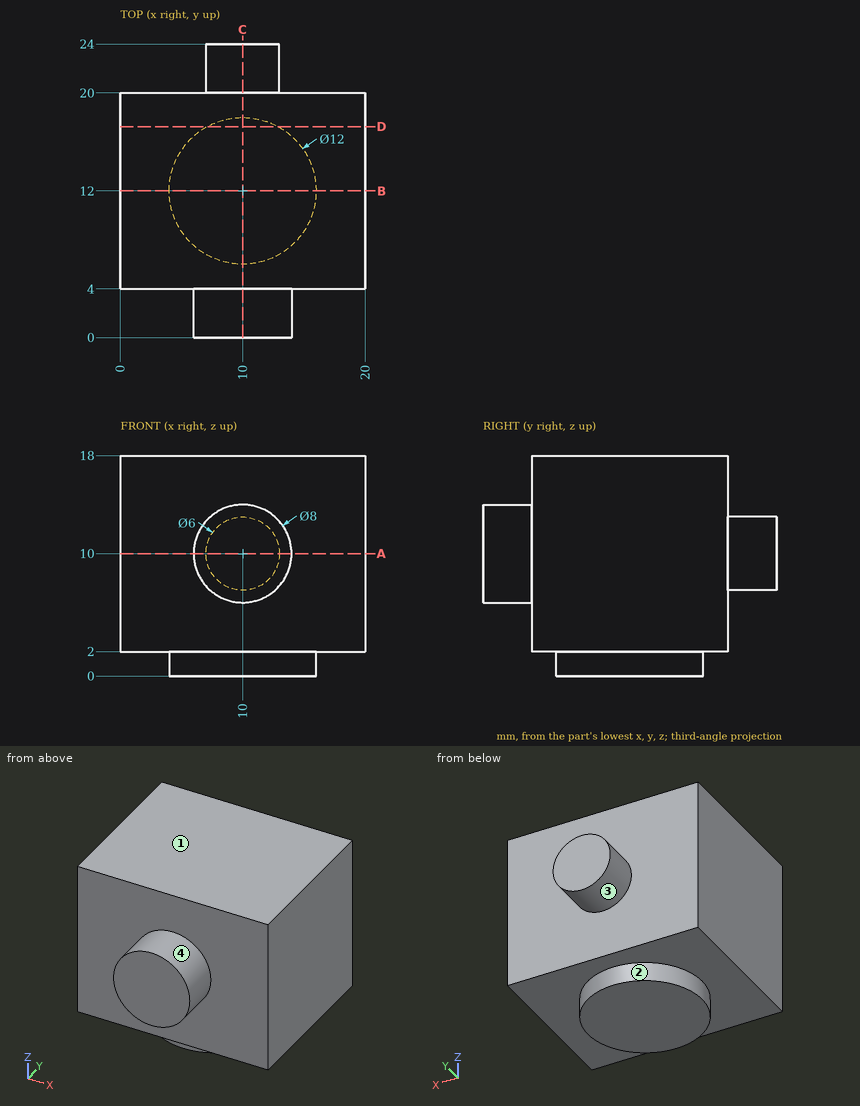
Design review of the part shown in the three views and the two pictorial views. Dimensions are in mm from the part's minimum x, y and z. A direction names the side the tool comes from. Coordinates: 2 decimals unless noted, no trailing zeros. Loops run counter-clockwise (first coordinate to the right, second up) from the corner with the lowest first, then second, coordinate; pieces in that order, holes last.
Q1. Tool access review of the marked faces 1, 2, 3 and 4: name each direction out of +Z, -Z, +X, -X, +Y, -Y from which nothing blocks a thin tool from reaching the whole face with its end or side.
Reported:
face 1: +Z, +X, -X, +Y, -Y
face 2: -Z
face 3: +Y
face 4: -Y
Q2. For pin 1 (4 mm diameter, centred on x = 9.5, z = 2, fed in from +Y), flat-tipped, find the tip position at first contact; note if it passes through.
Reported:
pin 1: stops at y = 20
Q3. We need section A-A on z = 10. State the section outline as (x, y) points.
Reported:
outline: (0, 4) - (6, 4) - (6, 0) - (14, 0) - (14, 4) - (20, 4) - (20, 20) - (13, 20) - (13, 24) - (7, 24) - (7, 20) - (0, 20) - close
Q4. We need section B-B on y = 12. State the section outline as (x, z) points, and give its area (3 significant figures).
Reported:
outline: (0, 2) - (4, 2) - (4, 0) - (16, 0) - (16, 2) - (20, 2) - (20, 18) - (0, 18) - close
area: 344 mm2
Q5. We need section D-D on y = 17.25. State the section outline as (x, z) points.
Reported:
outline: (0, 2) - (7.1, 2) - (7.1, 0) - (12.9, 0) - (12.9, 2) - (20, 2) - (20, 18) - (0, 18) - close
Q6. To check wall thickness, follow line 1 (Y direction, x = 17.75, z = 12.5); line 2 (Y direction, x = 10.5, z = 13.75); line 3 (Z direction, x = 2, y = 16.5). State the ranges of each line that lie inside material, in increasing order.
Reported:
line 1: y = 4 to 20
line 2: y = 0 to 20
line 3: z = 2 to 18
Q7. We need section C-C on x = 10. State the section outline as (y, z) points, and give its area (3 significant figures).
Reported:
outline: (0, 6) - (4, 6) - (4, 2) - (6, 2) - (6, 0) - (18, 0) - (18, 2) - (20, 2) - (20, 7) - (24, 7) - (24, 13) - (20, 13) - (20, 18) - (4, 18) - (4, 14) - (0, 14) - close
area: 336 mm2
